Here's how the part is built. I have some questions about the finished solid (model axes, mm). A direction names the side the tool comes from. Give positions to 0.01 mm unless a question says otherwise; leave off trailing zeros. Use a Markdown table: item, result.
Autodesk Inventor part; units mm, degrees
ref_plane "YZ Plane" through (0, 0, 0) normal (1, 0, 0) x (0, 1, 0)
ref_plane "XZ Plane" through (0, 0, 0) normal (0, 1, 0) x (-1, 0, 0)
ref_plane "XY Plane" through (0, 0, 0) normal (0, 0, 1) x (1, 0, 0)
sketch "スケッチ1" plane through (0, 0, 0) normal (1, 0, 0) x (0, 1, 0)
  line L0 (0, 0) -> (20, 0)
  line L1 (20, 0) -> (20, -3.5)
  line L2 (20, -3.5) -> (22, -3.5)
  line L3 (22, -3.5) -> (22, -12.5)
  line L4 (22, -12.5) -> (0, -12.5)
  line L5 (0, -12.5) -> (0, 0)
  line L6 (12, 0) -> (12, -12.5)
  dimension "d0" = 20
  dimension "d1" = 2
  dimension "d23" = 12
  dimension "d35" = 3.5
  dimension "d40" = 9
revolve "回転1" add sketch "スケッチ1" angle 360 about axis through (0, 0, -12.5) along (0, 0, 1)
chamfer "面取り1" distance 0.5 angle 45 1 edges at (0, -20, 0)
sketch "スケッチ4" plane through (0, 0, -12.5) normal (0, 0, -1) x (-1, 0, 0)
  circle A0 centre (0, 0) radius 15
  point P0 (0, 15)
  point P1 (-10.6066, 10.6066)
  point P2 (-15, 0)
  point P3 (-10.6066, -10.6066)
  point P4 (0, -15)
  point P5 (10.6066, -10.6066)
  point P6 (15, 0)
  point P7 (10.6066, 10.6066)
  dimension "d41" = 30
  dimension "d44" = 360
hole "穴2" at (-10.6066, 10.6066, -12.5) at (-15, 0, -12.5) at (-10.6066, -10.6066, -12.5) at (0, -15, -12.5) at (10.6066, -10.6066, -12.5) at (15, 0, -12.5) at (10.6066, 10.6066, -12.5) at (0, 15, -12.5) direction (0, 0, 1) diameter 4.3 end through all counterbore diameter 8 counterbore depth 2
sketch "スケッチ6" plane through (0, 0, 0) normal (0, 0, 1) x (1, 0, 0)
  circle A0 centre (0, 0) radius 7.6
  point P0 (0, 0)
  dimension "d46" = 15.2
extrude "押し出し3" cut sketch "スケッチ6" against normal blind 6.5
sketch "スケッチ7" plane through (0, 0, -6.5) normal (0, 0, 1) x (1, 0, 0)
  circle A0 centre (0, 0) radius 6
  point P0 (0, 0)
  dimension "d49" = 12
extrude "押し出し4" cut sketch "スケッチ7" against normal through all
properties part number "scara-base16" material "ABS プラスチック"
Item 1: Thinking about a two-plate mould opening in X: for faces 1 (the cylindrical face through (-19.524, -4.336, -2.021)), 2 (the flat face through (2, -13, -10.5)), 3 (the flat face through (5, 5, -12.5)), 4 (the flat face through (2, 17, -10.5)), which applies, +X half, -X half, draft (parallel to the pull), parting line (faces both ways), or undercut?
Values:
| item | result |
|---|---|
| face 1 | parting line |
| face 2 | undercut |
| face 3 | draft |
| face 4 | undercut |
Item 2: Will these pins go through, and if not, where does the flat tip stop? pin 1 Ø4 at (x, y) = (16, 0.5) entering from -Z; pin 2 Ø1 at (x, z) = (-4.5, -10.5) entering from -Y; pin 3 Ø2 at (y, z) = (9.5, -9) entering from -X; pin 4 Ø4 at (x, y) = (10.61, -10.61) entering from -Z.
Values:
| item | result |
|---|---|
| pin 1 | stops at z = -10.5 |
| pin 2 | stops at y = -21.63 |
| pin 3 | stops at x = -20.29 |
| pin 4 | passes through |
Item 3: If we section it at A-A, the plane y = 0: Count the separate pieces of the cut face and the enclosed holes in it, plus the area to 3 significant figures.
Values:
| item | result |
|---|---|
| separate pieces | 4 |
| enclosed holes | 0 |
| area | 243 mm2 |
Item 4: I need wall thicknesses on line 1 along Y through (x, z) = (0, -8); line 2 along Z through (x, y) = (-9, 9); line 3 along Z through (x, y) = (19.5, 5). Which ranges of each line are inside material? Lowest first, please. Write a range as [from, to].
Values:
| item | result |
|---|---|
| line 1 | y = [-22, -17.15], [-12.85, -6], [6, 12.85], [17.15, 22] |
| line 2 | z = [-10.5, 0] |
| line 3 | z = [-12.5, -3.5] |
Item 5: For faces 5 (the cylindrical face through (-0.65, 17.05, -5.18)), 6 (the cylindrical face through (-7.593, 0.334, -3.204)), 7 (the cylindrical face through (0, -19, -11)), which set-ups out of +Z, -Z, +X, -X, +Y, -Y let a thin tool reach every point of the face, with its end or its side?
Values:
| item | result |
|---|---|
| face 5 | +Z, -Z |
| face 6 | +Z |
| face 7 | -Z |
